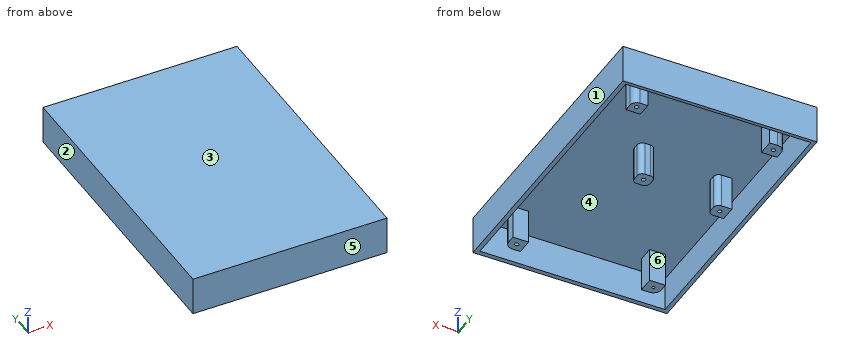
from build123d import *

# Parameters (mm, degrees)
SKETCH002_W   = 95
SKETCH002_H   = 140
PAD_DEPTH     = 2
SKETCH001_W   = 95
SKETCH001_H   = 140
SKETCH001_W_2 = 90.742981
SKETCH001_H_2 = 136.114502
SKETCH001_R   = 1
SKETCH001_R_2 = 0.7
PAD001_DEPTH  = 16.7


with BuildPart() as part:
    # Sketch002 → Pad (new body)
    with BuildSketch(Plane.XY):
        Rectangle(SKETCH002_W, SKETCH002_H)
    extrude(amount=PAD_DEPTH)

    # Sketch001 → Pad001 (join)
    with BuildSketch(Plane.XY):
        Rectangle(SKETCH001_W, SKETCH001_H)
        with Locations((-0.042641, 0.300621)):
            Rectangle(SKETCH001_W_2, SKETCH001_H_2, mode=Mode.SUBTRACT)
        with BuildLine():
            ThreePointArc((-33.5, 59.835), (-36.222361, 58.707361), (-37.35, 55.985))
            Line((-37.35, 55.985), (-37.35, 52.135))
            Line((-37.35, 52.135), (-29.65, 52.135))
            Line((-29.65, 52.135), (-29.65, 59.835))
            Line((-29.65, 59.835), (-33.5, 59.835))
        make_face()
        with Locations((-33.5, 55.985)):
            Circle(SKETCH001_R, mode=Mode.SUBTRACT)
        with BuildLine():
            ThreePointArc((36.65, 55.985), (35.727386, 58.212386), (33.5, 59.135))
            Line((33.5, 59.135), (29.65, 59.135))
            Line((29.65, 59.135), (29.65, 52.135))
            Line((29.65, 52.135), (36.65, 52.135))
            Line((36.65, 52.135), (36.65, 55.985))
        make_face()
        with Locations((33.5, 55.985)):
            Circle(SKETCH001_R, mode=Mode.SUBTRACT)
        with BuildLine():
            Line((37.35, -52.135), (29.65, -52.135))
            Line((29.65, -52.135), (29.65, -59.835))
            Line((29.65, -59.835), (33.5, -59.835))
            ThreePointArc((33.5, -59.835), (36.222361, -58.707361), (37.35, -55.985))
            Line((37.35, -55.985), (37.35, -52.135))
        make_face()
        with Locations((33.5, -55.985)):
            Circle(SKETCH001_R, mode=Mode.SUBTRACT)
        with BuildLine():
            Line((-33.5, -59.835), (-29.65, -59.835))
            Line((-29.65, -59.835), (-29.65, -52.135))
            Line((-29.65, -52.135), (-37.35, -52.135))
            Line((-37.35, -55.985), (-37.35, -52.135))
            ThreePointArc((-37.35, -55.985), (-36.222361, -58.707361), (-33.5, -59.835))
        make_face()
        with Locations((-33.5, -55.985)):
            Circle(SKETCH001_R_2, mode=Mode.SUBTRACT)
        with BuildLine():
            ThreePointArc((-29.65, 7.328333), (-30.401759, 9.143241), (-32.216667, 9.895))
            Line((-37.35, 9.895), (-32.216667, 9.895))
            Line((-37.35, 2.195), (-37.35, 9.895))
            Line((-32.216667, 2.195), (-37.35, 2.195))
            ThreePointArc((-32.216667, 2.195), (-30.401759, 2.946759), (-29.65, 4.761667))
            Line((-29.65, 7.328333), (-29.65, 4.761667))
        make_face()
        with Locations((-33.5, 6.045)):
            Circle(SKETCH001_R, mode=Mode.SUBTRACT)
        with BuildLine():
            Line((2.586847, 12.222931), (2.586847, 9.656265))
            ThreePointArc((2.586847, 9.656265), (3.338606, 7.841357), (5.153514, 7.089598))
            Line((5.153514, 7.089598), (7.72018, 7.089598))
            ThreePointArc((7.72018, 7.089598), (9.535088, 7.841357), (10.286847, 9.656265))
            Line((10.286847, 9.656265), (10.286847, 12.222931))
            ThreePointArc((10.286847, 12.222931), (9.535088, 14.037839), (7.72018, 14.789598))
            Line((7.72018, 14.789598), (5.153514, 14.789598))
            ThreePointArc((5.153514, 14.789598), (3.338606, 14.037839), (2.586847, 12.222931))
        make_face()
        with Locations((6.436847, 10.939598)):
            Circle(SKETCH001_R, mode=Mode.SUBTRACT)
    extrude(amount=-PAD001_DEPTH)


solid = part.part
The listing builds one solid part. Answer for the finished solid, in the listing's coordinates (mm). Face numbers are marked on the shaded views. A direction names the side the tool comes from. Coordinates: 2 decimals unless noted, no trailing zeros. Write each loop counter-clockwise with the first axis right and the second up, starting at its lowest first coordinate (ties: lowest second). Pieces come first, ordered by that corner, then holes. Notation, with made-up numbers: (-25.5, -13.75) - (1.5, -13.75) arc R5 ccw to (1.5, -5.75) - close; hole circle Ø6 at (85, 69.5). An arc over 180 degrees is marked (long way). Answer as CSV lines item,"result".
1. Given P1, Ø1, axis at x = 24, y = 49.5, coming from the -Z side, flat-ended and moving along its own axis, determine where the tip first touches the part or whether it passes through.
Computed values:
P1,"stops at z = 0"
2. Find section A-A (x = -9.5). Give the vertices of the cut face in (y, z), plus the area to 3 significant figures.
Computed values:
outline,"(-70, -16.7) - (-67.76, -16.7) - (-67.76, 0) - (68.36, 0) - (68.36, -16.7) - (70, -16.7) - (70, 2) - (-70, 2) - close"
area,"345 mm²"
3. Straight lines are drawn through the part: line 1 (Y direction, x = 33.5, z = -8.75) (3 decimals); line 2 (Y direction, x = -18, z = -13.5); line 3 (X direction, y = -60.5, z = -6.75). For each, find the intervals that lie inside material, in ascending order. Write a range as [from, to].
Computed values:
line 1,"y = [-70, -67.757], [-59.835, -56.985], [-54.985, -52.135], [52.135, 54.985], [56.985, 59.135], [68.358, 70]"
line 2,"y = [-70, -67.76], [68.36, 70]"
line 3,"x = [-47.5, -45.41], [45.33, 47.5]"
4. Find section B-B (z = -3.25). Give the number of separate pieces and of enclosed holes in the cut face, plus the area to 3 significant figures.
Computed values:
separate pieces,"7"
enclosed holes,"7"
area,"1,260 mm²"
5. A tool of negligible diameter and unlimited length cuts with its end or side. For the marked faces 5 and 6, from which of +Z, -Z, +X, -X, +Y, -Y can it reach the whole face along a straight path? Write none if from no direction.
Computed values:
face 5,"+Z, -Z, +X, -X, -Y"
face 6,"-Z"
6. Determine the mould class of the marked faces 1, 2, 3 and 4 for opening direction X: +X half, -X half, draft (parallel to the pull), parting line (faces both ways), or undercut.
Computed values:
face 1,"+X half"
face 2,"-X half"
face 3,"draft"
face 4,"undercut"
